from build123d import *

# Parameters (mm, degrees)
F1_DEPTH = 69
F2_R     = 5
F3_SIZE  = 5
F4_R     = 20.707169
F5_DEPTH = 69
F6_SIZE  = 5


with BuildPart() as f1:
    # F0 (on Front) → F1 (new body)
    with BuildSketch(Plane.XZ):
        with BuildLine():
            Line((-46.385089, -46.113969), (-46.385089, -96.113969))
            Line((-46.385089, -96.113969), (-46.385089, -146.113969))
            Line((-46.385089, -146.113969), (3.614911, -121.113969))
            Line((3.614911, -121.113969), (53.614911, -146.113969))
            Line((53.614911, -146.113969), (53.614911, -96.113969))
            ThreePointArc((53.614911, -96.113969), (38.97025, -60.75863), (3.614911, -46.113969))
            Line((3.614911, -46.113969), (-46.385089, -46.113969))
        make_face()
    extrude(amount=-F1_DEPTH)

    # F2
    f2_edges = [f1.edges().sort_by_distance(p)[0] for p in [
        (-21.385089, 69, -46.113969),
        (-46.385089, 69, -96.113969),
        (-21.385089, 69, -133.613969),
        (28.614911, 69, -133.613969),
        (53.614911, 69, -121.113969),
        (38.97025, 69, -60.75863),
    ]]
    fillet(f2_edges, radius=F2_R)

    # F3
    f3_edges = [f1.edges().sort_by_distance(p)[0] for p in [
        (-21.385089, 0, -46.113969),
        (-46.385089, 0, -96.113969),
        (-21.385089, 0, -133.613969),
        (28.614911, 0, -133.613969),
        (53.614911, 0, -121.113969),
        (38.97025, 0, -60.75863),
    ]]
    chamfer(f3_edges, length=F3_SIZE)

    # F4 (on face) → F5 (cut)
    with BuildSketch(Plane.XZ):
        with Locations((0, -84.683239)):
            Circle(F4_R)
    extrude(amount=-F5_DEPTH, mode=Mode.SUBTRACT)

    # F6
    f6_edges = [f1.edges().sort_by_distance(p)[0] for p in [
        (20.707169, 34.5, -84.683239),
        (-20.707169, 0, -84.683239),
        (-20.707169, 69, -84.683239),
    ]]
    chamfer(f6_edges, length=F6_SIZE)


solid = f1.part
Geometry check sheet. Reference: the model listing, model coordinates, mm. A direction names the side the tool comes from. Round coordinates to 2 decimals unless told otherwise and drop trailing zeros. Order: outer loops, then holes, each group sorted by start corner. A loop starts at its lowest first (then second) coordinate and runs counter-clockwise, first axis right, second up. Notation, with made-up numbers: M -6,25.25 L 25,25.25 A22 ccw 25,64.25 Z; hole C -25.75,3.5 d7. An arc over 180 degrees is marked long. Answer in a Markdown table with one row per item.
(1) Tool access check on faces 4 (the face through (-21.74, 34.09, -133.79)), 5 (the face through (28.23, 2.54, -130.67)), 6 (the face through (-4.5, 64.2, -105.1)), 7 (the face through (28.5, 67.5, -131.96)). Record the directions out of +Z, -Z, +X, -X, +Y, -Y that give a thin tool (end or side, any length) a straight path to the whole face; none if there is none.
Responses:
| item | result |
|---|---|
| face 4 | -Z, +Y, -Y |
| face 5 | -Z, -Y |
| face 6 | +Y |
| face 7 | -Z, +Y |
(2) Scan lines: probe 1 along X at (y, z) = (60.5, -66); probe 2 along Z at (x, y) = (-16.5, 16); probe 3 along X at (y, z) = (9, -102). Record each from-to range of solid material in increasing order. Write a range as from..to.
Responses:
| item | result |
|---|---|
| probe 1 | x = -46.39..-8.93, 8.93..43.53 |
| probe 2 | z = -131.17..-97.19, -72.17..-46.11 |
| probe 3 | x = -46.39..-11.35, 11.35..53.61 |
(3) Draft check along X on faces 1 (the face through (-21.735, 67.496, -47.54)), 2 (the face through (-46.385, 34, -95)), 3 (the face through (-21.735, 2.535, -131.033)). Enter one of: released by +X, released by -X, zero draft, split by the parting line, or undercut.
Responses:
| item | result |
|---|---|
| face 1 | zero draft |
| face 2 | released by -X |
| face 3 | undercut |
(4) Go/stop test with flat-tipped pins: P1, Ø10, axis at x = -20.5, y = 53, coming from the -Z side; P2, Ø10, axis at x = -27, y = 45.5, coming from the -Z side; P3, Ø1, axis at x = 32.5, y = 45, coming from the +Z side. Record where each tip stops, or that it passes through.
Responses:
| item | result |
|---|---|
| P1 | stops at z = -135.67 |
| P2 | stops at z = -138.92 |
| P3 | stops at z = -54.95 |
(5) Sectioned sample at A-A, the plane y = 34. Record the cut outline in (x, z), and give its area (3 significant figures).
Responses:
| item | result |
|---|---|
| outline | M -46.39,-146.11 L 3.61,-121.11 L 53.61,-146.11 L 53.61,-96.11 A50 ccw 3.61,-46.11 L -46.39,-46.11 Z; hole C 0,-84.68 d41.41 |
| area | 6,870 mm² |
